CAD build for the part. Positions are in the model's coordinates, mm. Coordinates: 2 decimals unless noted, no trailing zeros. Write each loop counter-clockwise with the first axis right and the second up, starting at its lowest first coordinate (ties: lowest second). Pieces come first, ordered by that corner, then holes. Notation, with made-up numbers: (28, 22) - (60, 22) arc R20 cw to (60, 36) - close; hole circle Ø11 at (58, -20). An arc over 180 degrees is marked (long way). Answer in a Markdown table with one row per item. Add a question column.
Q1. Band-saw the part on D-D (y = 31). List the corners of the cut face in (x, z), and give its area (3 significant figures).
Q2. Band-saw the part on C-C (z = -30). List the corners of the cut face in (x, y).
Q3. Pin check, flat tips, straight feed: pin 1 (12 mm diameter, centred on x = -162.5, y = 18.5, fed in from -Z); pin 2 (3 mm diameter, centred on x = -110.5, z = -2.5, fed in from -Y). Stop position of each tip, or through.
Q4. Band-saw the part on B-B (y = -76.2). List the corners of the cut face in (x, z).
Q5. Drill centre lines: line 1 along X through (y, z) = (-72, -22.5); line 2 along Z through (x, y) = (258, 79); line 3 along X through (y, z) = (-73, -28). Where is each one in solid material? Low to high. Write a range as from..to.
Q6. Band-saw the part on A-A (x = 0). List the corners of the cut face in (y, z).
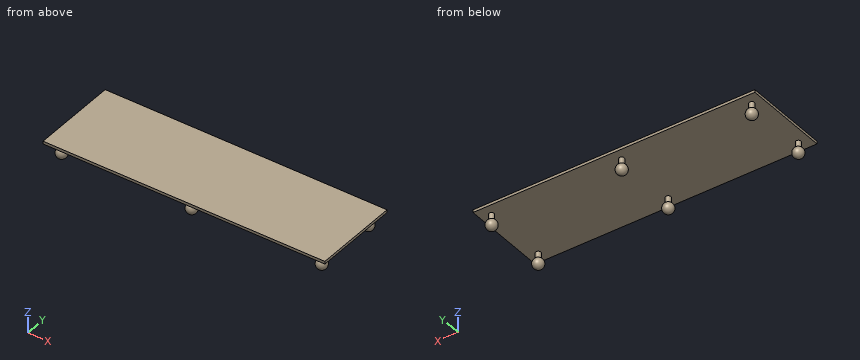
```python
from build123d import *

# Parameters (mm, degrees)
SKETCH1_W           = 660.4
SKETCH1_H           = 203.2
BOSS_EXTRUDE1_DEPTH = 6.35
LPATTERN1_COUNT     = 2
LPATTERN1_PITCH     = 304.8
LPATTERN1_COL_COUNT = 2
LPATTERN1_COL_PITCH = 304.8


with BuildPart() as part:
    # Sketch1 → Boss-Extrude1 (new body)
    with BuildSketch(Plane.XY):
        Rectangle(SKETCH1_W, SKETCH1_H)
    extrude(amount=BOSS_EXTRUDE1_DEPTH)

    # Sketch3 → Revolve1 (revolve)
    with BuildSketch(Plane(origin=(0, 0, 0), x_dir=(0, 0, -1), z_dir=(1, 0, 0))):
        with BuildLine():
            Line((0, -76.2), (38.1, -76.2))
            ThreePointArc((38.1, -76.2), (28.44332506, -88.529970502), (14.158555499, -82.10930838))
            Line((14.158555499, -82.10930838), (0, -82.10930838))
            Line((0, -82.10930838), (0, -76.2))
        make_face()
    revolve1 = revolve(axis=Axis((0, -76.2, 0), (0, 0, -1)))

    # Mirror1: Revolve1 across plane
    add(revolve1.mirror(Plane.ZX))

    # LPattern1: Revolve1 ×2
    with Locations(*[(i * LPATTERN1_PITCH, 0, 0) for i in range(1, LPATTERN1_COUNT)]):
        add(revolve1)

    # LPattern1 copy 1 sketch → LPattern1 copy 1 (revolve)
    with BuildSketch(Plane(origin=(304.8, 0, 0), x_dir=(0, 0, -1), z_dir=(1, 0, 0))):
        with BuildLine():
            Line((0, 76.2), (38.1, 76.2))
            ThreePointArc((38.1, 76.2), (28.44332506, 88.529970502), (14.158555499, 82.10930838))
            Line((14.158555499, 82.10930838), (0, 82.10930838))
            Line((0, 82.10930838), (0, 76.2))
        make_face()
    revolve(axis=Axis((304.8, 76.2, 0), (0, 0, 1)))

    # LPattern1 col: Revolve1 ×2
    with Locations(*[(-i * LPATTERN1_COL_PITCH, 0, 0) for i in range(1, LPATTERN1_COL_COUNT)]):
        add(revolve1)

    # LPattern1 col copy 1 sketch → LPattern1 col copy 1 (revolve)
    with BuildSketch(Plane(origin=(-304.8, 0, 0), x_dir=(0, 0, -1), z_dir=(1, 0, 0))):
        with BuildLine():
            Line((0, 76.2), (38.1, 76.2))
            ThreePointArc((38.1, 76.2), (28.44332506, 88.529970502), (14.158555499, 82.10930838))
            Line((14.158555499, 82.10930838), (0, 82.10930838))
            Line((0, 82.10930838), (0, 76.2))
        make_face()
    revolve(axis=Axis((-304.8, 76.2, 0), (0, 0, 1)))


solid = part.part
```
Checked values:
| question | item | result |
|---|---|---|
| 1 | outline | (-330.2, 0) - (330.2, 0) - (330.2, 6.35) - (-330.2, 6.35) - close |
| 1 | area | 4,190 mm² |
| 2 | outline | circle Ø23.68 at (-304.8, -76.2); circle Ø23.68 at (-304.8, 76.2); circle Ø23.68 at (0, -76.2); circle Ø23.68 at (0, 76.2); circle Ø23.68 at (304.8, -76.2); circle Ø23.68 at (304.8, 76.2) |
| 3 | pin 1 | stops at z = 0 |
| 3 | pin 2 | passes through |
| 4 | outline | (-330.2, 0) - (-310.71, 0) - (-310.71, -14.16) arc R12.7 ccw (long way) to (-298.89, -14.16) - (-298.89, 0) - (-5.91, 0) - (-5.91, -14.16) arc R12.7 ccw (long way) to (5.91, -14.16) - (5.91, 0) - (298.89, 0) - (298.89, -14.16) arc R12.7 ccw (long way) to (310.71, -14.16) - (310.71, 0) - (330.2, 0) - (330.2, 6.35) - (-330.2, 6.35) - close |
| 5 | line 1 | x = -316.43..-293.17, -11.63..11.63, 293.17..316.43 |
| 5 | line 2 | z = 0..6.35 |
| 5 | line 3 | x = -316.81..-292.79, -12.01..12.01, 292.79..316.81 |
| 6 | outline | (-101.6, 0) - (-82.11, 0) - (-82.11, -14.16) arc R12.7 ccw (long way) to (-70.29, -14.16) - (-70.29, 0) - (70.29, 0) - (70.29, -14.16) arc R12.7 ccw (long way) to (82.11, -14.16) - (82.11, 0) - (101.6, 0) - (101.6, 6.35) - (-101.6, 6.35) - close |
